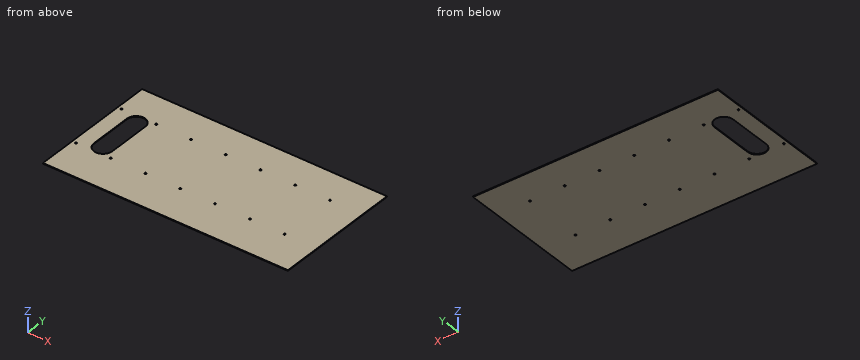
```python
from build123d import *

# Parameters (mm, degrees)
SKETCH1_W                = 506
SKETCH1_H                = 267.33784
BASE_FLANGE1_DEPTH       = 1.51892
CUT_EXTRUDE1_DEPTH       = 2.54
M3_CLEARANCE_HOLE1_D     = 3.6
M3_CLEARANCE_HOLE1_DEPTH = 11.938
M3_CLEARANCE_HOLE1_TIP   = 1.081549114


# Sheet-metal steps are written as plain solids
with BuildPart() as part:
    # Sketch1 → Base-Flange1 (new body)
    with BuildSketch(Plane.XY):
        with Locations((-172.1425, 68.65)):
            Rectangle(SKETCH1_W, SKETCH1_H)
    extrude(amount=BASE_FLANGE1_DEPTH)

    # Sketch6 → Cut-Extrude1 (cut)
    with BuildSketch(Plane.XY.offset(1.51892)):
        with BuildLine():
            Line((-393.3925, 30.86892), (-393.3925, 119.76892))
            ThreePointArc((-393.3925, 119.76892), (-374.3425, 138.81892), (-355.2925, 119.76892))
            Line((-355.2925, 119.76892), (-355.2925, 30.86892))
            ThreePointArc((-355.2925, 30.86892), (-374.3425, 11.81892), (-393.3925, 30.86892))
        make_face()
    extrude(amount=-CUT_EXTRUDE1_DEPTH, mode=Mode.SUBTRACT)

    # M3 Clearance Hole1
    with Locations(Plane.XY.offset(1.51892)):
        with Locations((-417.1425, 136.3375), (-417.1425, 13.6625), (-345.341667, 136.3375), (-345.341667, 13.6625), (-273.540834, 136.3375), (-273.540834, 13.6625), (-201.740001, 136.3375), (-201.740001, 13.6625), (-129.939168, 136.3375), (-129.939168, 13.6625), (-58.138335, 136.3375), (-58.138335, 13.6625), (13.662498, 136.3375), (13.662498, 13.6625)):
            Hole(M3_CLEARANCE_HOLE1_D / 2, depth=M3_CLEARANCE_HOLE1_DEPTH)
            with Locations((0, 0, -(M3_CLEARANCE_HOLE1_DEPTH + M3_CLEARANCE_HOLE1_TIP / 2))):  # 118° drill point
                Cone(0, M3_CLEARANCE_HOLE1_D / 2, M3_CLEARANCE_HOLE1_TIP, mode=Mode.SUBTRACT)


solid = part.part
```
Input: part model. Units: mm. Frame: model coordinates. Give positions to 0.01 mm unless a question says otherwise; leave off trailing zeros. Order: outer loops, then holes, each group sorted by start corner. A loop starts at its lowest first (then second) coordinate and runs counter-clockwise, first axis right, second up. Notation, with made-up numbers: M 22.5,-6.75 L 26.5,-6.75 A7 cw 26.5,0.25 Z; hole C 16.5,-15.5 d6. An arc over 180 degrees is marked long. One line per question, with ' | ' between items. Start each with the question number.
1. Section query B-B (z = 1.2). Count the separate pieces of the cut face and the enclosed holes in it, and give its area (3 significant figures).
2. Material intervals for probe 1 along Y at (x, z) = (-201.74, 0.4); probe 2 along X at (y, z) = (82, 1.3); probe 3 along Y at (x, z) = (-391.5, 0.3), sorted ascending. Write a range as [from, to].
3. Section query A-A (y = 84). Return the cut outline in (x, z).
Here are the results:
1) separate pieces: 1 | enclosed holes: 15 | area: 131,000 mm²
2) probe 1: [-65.02, 11.86], [15.46, 134.54], [138.14, 202.32] | probe 2: [-425.14, -393.39], [-355.29, 80.86] | probe 3: [-65.02, 22.59], [128.05, 202.32]
3) outline: M -425.14,0 L -393.39,0 L -393.39,1.52 L -425.14,1.52 Z; M -355.29,0 L 80.86,0 L 80.86,1.52 L -355.29,1.52 Z
